Input: part model. Units: mm. Frame: model coordinates. A direction names the side the tool comes from. Coordinates: 2 decimals unless noted, no trailing zeros. Order: outer loops, then holes, each group sorted by start corner. A loop starts at its lowest first (then second) coordinate and runs counter-clockwise, first axis right, second up. Notation, with made-up numbers: (34.5, 75.5) - (81.5, 75.5) arc R20 ccw to (81.5, 86.5) - close; hole circle Ø10 at (23, -8). An arc over 180 degrees is marked (long way). Use a Markdown table: item, result. Add a question column.
from build123d import *
from OCP.BRepFilletAPI import BRepFilletAPI_MakeChamfer

# Parameters (mm, degrees)
EXTRUDE_1_DEPTH     = 131
EXTRUDE_2_DEPTH     = 116
CUT_EXTRUDE_1_REACH = 148.45
CUT_EXTRUDE_2_REACH = 148.994
EXTRUDE_3_DEPTH     = 134
CUT_EXTRUDE_3_DEPTH = 67
EXTRUDE_4_DEPTH     = 11
EXTRUDE_START       = -33.5
EXTRUDE_5_DEPTH     = 67
EXTRUDE_6_DEPTH     = 2
EXTRUDE_7_DEPTH     = 20
EXTRUDE_8_DEPTH     = 10
EXTRUDE_9_DEPTH     = 10
CUT_EXTRUDE_4_REACH = 246.491
SKETCH_16_W         = 5.440253517
SKETCH_16_H         = 47
CUT_EXTRUDE_5_DEPTH = 219.790404517
EXTRUDE_10_DEPTH    = 15
CUT_EXTRUDE_6_DEPTH = 15
EXTRUDE_15_DEPTH    = 77
SKETCH_23_R         = 7
SKETCH_23_R_2       = 4.5
EXTRUDE_16_DEPTH    = 3
CHAMFER_1_SIZE      = 3
CHAMFER_1_SIZE_2    = 1.732050808
CHAMFER_2_SIZE      = 3
CHAMFER_2_SIZE2     = 1.907428497


# Read off the part's stored shape, not the designer's step: 凸台-拉伸5
with BuildPart() as part:
    # 草图1 → 凸台-拉伸1 (new body)
    with BuildSketch(Plane.XY):
        Polygon((0, 0), (3, 20), (39, 20), (42, 0), (39, -35), (3, -35), align=None)
    extrude(amount=-EXTRUDE_1_DEPTH)

    # 草图2 → 凸台-拉伸2 (add)
    with BuildSketch(Plane.XY.offset(-15)):
        Polygon((-2, 24.7), (-4.8, 0.2), (-4.8, -5.8), (-2, -40.3), (21, -40.3), (21, -35), (3, -35), (0, 0), (3, 20), (21, 20), (21, 24.7), align=None)
        Polygon((44, 24.7), (21, 24.7), (21, 20), (39, 20), (42, 0), (39, -35), (21, -35), (21, -40.3), (44, -40.3), (46.8, -5.8), (46.8, 0.2), align=None)
    extrude(amount=-EXTRUDE_2_DEPTH)

    # 切除-拉伸1: up to this plane
    cut_extrude_1_end = Plane(origin=(3, -35, -131), z_dir=(-0.996346649041751, -0.08540114134643588, 0))
    # 草图3 → 切除-拉伸1 (cut, up to the surface)
    with BuildSketch(Plane.ZY.offset(4.8), mode=Mode.PRIVATE) as cut_extrude_1_sk1:
        Polygon((-131, -40.3), (-131, -10.092413278), (-95, -40.3), align=None)
    cut_extrude_1_tool1 = split(extrude(cut_extrude_1_sk1.sketch, amount=-CUT_EXTRUDE_1_REACH, mode=Mode.PRIVATE), bisect_by=cut_extrude_1_end, keep=Keep.BOTH, mode=Mode.PRIVATE)
    add(cut_extrude_1_tool1.solids().sort_by_distance((-4.8, -30.230804, -119))[0], mode=Mode.SUBTRACT)
    # 草图3 → 切除-拉伸1 (cut, up to the surface)
    with BuildSketch(Plane.ZY.offset(4.8), mode=Mode.PRIVATE) as cut_extrude_1_sk2:
        Polygon((-62, -40.3), (-30.5, -8.8), (-15, -8.8), (-15, -40.3), align=None)
    cut_extrude_1_tool2 = split(extrude(cut_extrude_1_sk2.sketch, amount=-CUT_EXTRUDE_1_REACH, mode=Mode.PRIVATE), bisect_by=cut_extrude_1_end, keep=Keep.BOTH, mode=Mode.PRIVATE)
    add(cut_extrude_1_tool2.solids().sort_by_distance((-4.8, -27.196, -31.948))[0], mode=Mode.SUBTRACT)

    # 切除-拉伸2: up to this plane
    cut_extrude_2_end = Plane(origin=(42, 0, -131), z_dir=(0.996346649041751, -0.08540114134643569, 0))
    # 草图4 → 切除-拉伸2 (cut, up to the surface)
    with BuildSketch(Plane(origin=(46.8, 0, 0), x_dir=(0, 0, -1), z_dir=(1, 0, 0)), mode=Mode.PRIVATE) as cut_extrude_2_sk1:
        Polygon((15, -8.919073988), (15, -40.419073988), (62, -40.419073988), (30.5, -8.919073988), align=None)
    cut_extrude_2_tool1 = split(extrude(cut_extrude_2_sk1.sketch, amount=CUT_EXTRUDE_2_REACH, dir=(-0.996346649042, 0.085401141346, 0), mode=Mode.PRIVATE), bisect_by=cut_extrude_2_end, keep=Keep.BOTH, mode=Mode.PRIVATE)
    add(cut_extrude_2_tool1.solids().sort_by_distance((46.8, -27.315074, -31.948))[0], mode=Mode.SUBTRACT)

    # 草图6 → 凸台-拉伸3 (add)
    with BuildSketch(Plane.XY.offset(-11)):
        Polygon((-9, 29.7), (1, 24.7), (41, 24.7), (51, 29.7), (51, 44.7), (41, 49.7), (1, 49.7), (-9, 44.7), align=None)
    extrude(amount=-EXTRUDE_3_DEPTH)

    # 草图7 → 切除-拉伸3 (cut, symmetric)
    with BuildSketch(Plane.ZY.offset(4.8)):
        Polygon((-95, -40.3), (-131, -40.3), (-131, -9.728583388), align=None)
        Polygon((-145, 24.7), (-135, 49.7), (-145, 49.7), align=None)
    extrude(amount=CUT_EXTRUDE_3_DEPTH, both=True, mode=Mode.SUBTRACT)

    # 草图9 → 凸台-拉伸4 (add)
    with BuildSketch(Plane.XY.offset(-11)):
        Polygon((3.5, 45.7), (3.5, 28.7), (8.5, 26.2), (33.5, 26.2), (38.5, 28.7), (38.5, 45.7), (33.5, 48.2), (8.5, 48.2), align=None)
    extrude(amount=EXTRUDE_4_DEPTH)

    # 凸台-拉伸5 outline → 凸台-拉伸5 (add)
    with BuildSketch(Plane.ZY.offset(-21).offset(EXTRUDE_START)):
        with BuildLine():
            Line((-118.5, 35.555969457), (-83.798221281, -5.8))
            ThreePointArc((-83.798221281, -5.8), (-66.915700425, -24.400324924), (-42.17780049, -20.038226285))
            ThreePointArc((-42.17780049, -20.038226285), (-40.182635106, -18.251941452), (-38.381793618, -16.269905038))
            ThreePointArc((-38.381793618, -16.269905038), (-34.014561818, -8.544330565), (-32.5, 0.2))
            Line((-32.5, 0.2), (-32.5, 54.2))
            Line((-32.5, 54.2), (-118.5, 54.2))
            Line((-118.5, 54.2), (-118.5, 35.555969457))
        make_face()
    extrude(amount=EXTRUDE_5_DEPTH)

    # 草图11 → 凸台-拉伸6 (add)
    with BuildSketch(Plane.ZY.offset(12.5)):
        with BuildLine():
            Line((-84.5, 9.7), (-96.804265564, 9.7))
            Line((-96.804265564, 9.7), (-83.798221281, -5.8))
            ThreePointArc((-83.798221281, -5.8), (-66.915700425, -24.400324924), (-42.17780049, -20.038226285))
            ThreePointArc((-42.17780049, -20.038226285), (-40.182635106, -18.251941452), (-38.381793618, -16.269905038))
            ThreePointArc((-38.381793618, -16.269905038), (-34.014561818, -8.544330565), (-32.5, 0.2))
            Line((-32.5, 0.2), (-32.5, 9.7))
            ThreePointArc((-32.5, 9.7), (-58.5, 35.7), (-84.5, 9.7))
        make_face()
    extrude_6 = extrude(amount=EXTRUDE_6_DEPTH)

    # 镜向1: 凸台-拉伸6 across plane
    add(extrude_6.mirror(Plane.ZY.offset(-21)))

    # 草图12 → 凸台-拉伸7 (add)
    with BuildSketch(Plane(origin=(0, 54.2, 0), x_dir=(1, 0, 0), z_dir=(0, 1, 0))):
        Polygon((21, 100), (-6.5, 100), (-6.5, 32.5), (48.5, 32.5), (48.5, 100), align=None)
    extrude(amount=EXTRUDE_7_DEPTH)

    # 草图13 → 凸台-拉伸8 (add)
    with BuildSketch(Plane.ZY.offset(6.5)):
        Polygon((-95, 62.2), (-99.448556281, 147.083510454), (-88.463631398, 147.659205973), (-84.015075118, 62.775695519), align=None)
    extrude(amount=EXTRUDE_8_DEPTH)

    # 草图14 → 凸台-拉伸9 (add)
    with BuildSketch(Plane(origin=(48.5, 0, 0), x_dir=(0, 0, -1), z_dir=(1, 0, 0))):
        Polygon((84.613797545, 74.2), (95.628893351, 74.2), (99.448556281, 147.083510454), (88.463631398, 147.659205973), align=None)
        Polygon((84.015075118, 62.775695519), (95, 62.2), (95.628893351, 74.2), (84.613797545, 74.2), align=None)
    extrude(amount=EXTRUDE_9_DEPTH)

    # 切除-拉伸4: up to this plane
    cut_extrude_4_end = Plane(origin=(-16.436947072, -34.998764239, 0), z_dir=(-0.08540114134643567, -0.996346649041751, 0))
    # 草图16 → 切除-拉伸4 (cut, up to the surface)
    with BuildSketch(Plane.XZ.offset(40.3), mode=Mode.PRIVATE) as cut_extrude_4_sk1:
        with Locations((41.279873241, -38.5)):
            Rectangle(SKETCH_16_W, SKETCH_16_H)
    cut_extrude_4_tool1 = split(extrude(cut_extrude_4_sk1.sketch, amount=-CUT_EXTRUDE_4_REACH, mode=Mode.PRIVATE), bisect_by=cut_extrude_4_end, keep=Keep.BOTH, mode=Mode.PRIVATE)
    add(cut_extrude_4_tool1.solids().sort_by_distance((41.279873, -40.3, -38.5))[0], mode=Mode.SUBTRACT)

    # 草图17 → 切除-拉伸5 (cut, through all)
    with BuildSketch(Plane.ZY.offset(12.5)):
        Polygon((-15, -40.3), (-15, -35), (-56.7, -35), (-62, -40.3), align=None)
    extrude(amount=-CUT_EXTRUDE_5_DEPTH, mode=Mode.SUBTRACT)

    # 草图18 → 凸台-拉伸10 (add)
    with BuildSketch(Plane.XY):
        with BuildLine():
            Line((16.069933514, -1.66230637), (18.041960108, -13.328973037))
            ThreePointArc((18.041960108, -13.328973037), (21, -15.828973037), (23.958039892, -13.328973037))
            Line((23.958039892, -13.328973037), (25.930066486, -1.66230637))
            ThreePointArc((25.930066486, -1.66230637), (21, 4.171026963), (16.069933514, -1.66230637))
        make_face()
    extrude(amount=EXTRUDE_10_DEPTH)

    # 草图20 → 切除-拉伸6 (cut)
    with BuildSketch(Plane.XY.offset(15)):
        with BuildLine():
            Line((17.055946811, -1.495639704), (19.027973406, -13.16230637))
            ThreePointArc((19.027973406, -13.16230637), (21, -14.828973037), (22.972026594, -13.16230637))
            Line((22.972026594, -13.16230637), (24.944053189, -1.495639704))
            ThreePointArc((24.944053189, -1.495639704), (21, 3.171026963), (17.055946811, -1.495639704))
        make_face()
    extrude(amount=-CUT_EXTRUDE_6_DEPTH, mode=Mode.SUBTRACT)

    # 草图21 → 凸台-拉伸15 (add)
    with BuildSketch(Plane.XY.offset(15)):
        with BuildLine():
            Line((13.111893623, -2.16230637), (15.083920217, -13.828973037))
            ThreePointArc((15.083920217, -13.828973037), (21, -18.828973037), (26.916079783, -13.828973037))
            Line((26.916079783, -13.828973037), (28.888106377, -2.16230637))
            ThreePointArc((28.888106377, -2.16230637), (21, 7.171026963), (13.111893623, -2.16230637))
        make_face()
    extrude(amount=EXTRUDE_15_DEPTH)

    # 草图23 → 凸台-拉伸16 (add)
    with BuildSketch(Plane.XY.offset(92)):
        with Locations((21, -0.828973037)):
            Circle(SKETCH_23_R)
        with Locations((21, -12.828973037)):
            Circle(SKETCH_23_R_2)
    extrude(amount=EXTRUDE_16_DEPTH)

    # 倒角1
    chamfer_1_edges_1 = [part.edges().sort_by_distance(p)[0] for p in [
        (14, -0.828973037, 95),
    ]]
    chamfer_1_side_1 = [part.faces().sort_by_distance(p)[0] for p in [
        (14, -0.828973037, 94.965358984),
    ]]
    chamfer_1_edges_2 = [part.edges().sort_by_distance(p)[0] for p in [
        (16.5, -12.828973037, 95),
    ]]
    chamfer_1_side_2 = [part.faces().sort_by_distance(p)[0] for p in [
        (16.5, -12.828973037, 94.965358984),
    ]]
    chamfer_1 = BRepFilletAPI_MakeChamfer(part.part.solid().wrapped)
    for e in chamfer_1_edges_1:
        chamfer_1.Add(CHAMFER_1_SIZE - 0.0001, CHAMFER_1_SIZE_2 - 0.0001, e.wrapped, chamfer_1_side_1[0].wrapped)
    for e in chamfer_1_edges_2:
        chamfer_1.Add(CHAMFER_1_SIZE - 0.0001, CHAMFER_1_SIZE_2 - 0.0001, e.wrapped, chamfer_1_side_2[0].wrapped)
    add(Compound.cast(chamfer_1.Shape()), mode=Mode.REPLACE)  # a hair under: the kernel refuses the full size

    # 倒角2: one chamfer whose edges measure the first distance from different faces: ONE call of the kernel's chamfer builder (chamfer() names one face for all edges)
    chamfer_2_edges_1 = [part.edges().sort_by_distance(p)[0] for p in [
        (3, -35, -28.35),
    ]]
    chamfer_2_side_1 = [part.faces().sort_by_distance(p)[0] for p in [
        (21, -35, -28.35),
    ]]
    chamfer_2_edges_2 = [part.edges().sort_by_distance(p)[0] for p in [
        (39, -35, -28.35),
    ]]
    chamfer_2_side_2 = [part.faces().sort_by_distance(p)[0] for p in [
        (40.177893681, -21.257907057, -21.206076587),
    ]]
    chamfer_2 = BRepFilletAPI_MakeChamfer(part.part.solid().wrapped)
    for e in chamfer_2_edges_1:
        chamfer_2.Add(CHAMFER_2_SIZE, CHAMFER_2_SIZE2, e.wrapped, chamfer_2_side_1[0].wrapped)  # the first distance lies on this face
    for e in chamfer_2_edges_2:
        chamfer_2.Add(CHAMFER_2_SIZE, CHAMFER_2_SIZE2, e.wrapped, chamfer_2_side_2[0].wrapped)  # the first distance lies on this face
    add(Compound.cast(chamfer_2.Shape()), mode=Mode.REPLACE)


solid = part.part
1) Pull-direction query (Y, two-part tool) for faces 5 (the flat face through (-12.5, 37, -76)), 6 (the flat face through (43.949, -8.675, -22.858)), 7 (the flat face through (21, 48.2, -6)); classes: pulls with the +Y half, pulls with the -Y half, needs draft (parallel to the pull), parting line crosses it, or undercut.
2) Material intervals for L1, parallel to Y at x = 7, z = -26; L2, parallel to Z at x = 27, y = 16; L3, parallel to Z at x = 40.5, y = 17, sorted ascending.
3) Cut plane A-A (y = 124). Return the cut outline in (x, z), and give its area (3 significant figures).
4) Cut plane B-B (z = 48). Return the cut outline in (x, y), and give its area (3 significant figures).
5) Contact query for flat-ended pins moving along their axis: P1, Ø10, axis at x = 9.5, y = 65.5, coming from the -Z side; P2, Ø12, axis at x = -8.5, y = -19, coming from the -Z side; P3, Ø22, axis at y = 63, z = -57.5, coming from the -X side. Output: stop coordinate, or through.
6) Cut plane C-C (y = 32.5). Return the cut outline in (x, z).
7) Reachability of faces 1 (the flat face through (46.07, 47.165, -21.6)), 2 (the flat face through (48.5, 111, -92)), 3 (the flat face through (-2, -8.8, -23)), 4 (the flat face through (21, 64, -100)) from +Z, -Z, +X, -X, +Y, -Y: full face, straight path, thin tool, end or side. Return the list, or none.
8) Cut plane D-D (z = -104). Return the cut outline in (x, y).
Computed:
| question | item | result |
|---|---|---|
| 1 | face 5 | undercut |
| 1 | face 6 | pulls with the -Y half |
| 1 | face 7 | pulls with the +Y half |
| 2 | L1 | y = -35 to 49.7 |
| 2 | L2 | z = -131 to 0 |
| 2 | L3 | z = -131 to -15 |
| 3 | outline | (-16.5, -98.24) - (-6.5, -98.24) - (-6.5, -87.22) - (-16.5, -87.22) - close; (48.5, -98.24) - (58.5, -98.24) - (58.5, -87.22) - (48.5, -87.22) - close |
| 3 | area | 220 mm2 |
| 4 | outline | (13.11, -2.16) - (15.08, -13.83) arc R6 ccw to (26.92, -13.83) - (28.89, -2.16) arc R8 ccw (long way) to start |
| 4 | area | 327 mm2 |
| 5 | P1 | stops at z = -100 |
| 5 | P2 | stops at z = -124.83 |
| 5 | P3 | stops at x = -12.5 |
| 6 | outline | (-14.5, -71) - (-12.5, -71) - (-12.5, -115.94) - (-9, -115.94) - (-9, -141.88) - (51, -141.88) - (51, -115.94) - (54.5, -115.94) - (54.5, -71) - (56.5, -71) - (56.5, -46) - (54.5, -46) - (54.5, -32.5) - (51, -32.5) - (51, -11) - (38.5, -11) - (38.5, 0) - (3.5, 0) - (3.5, -11) - (-9, -11) - (-9, -32.5) - (-12.5, -32.5) - (-12.5, -46) - (-14.5, -46) - close |
| 7 | face 1 | +Z, +X, +Y |
| 7 | face 2 | +Z, -Z, +Y |
| 7 | face 3 | +Z, -X, -Y |
| 7 | face 4 | -Z, +X, -X, +Y |
| 8 | outline | (-12.5, 18.28) - (-2.73, 18.28) - (-4.8, 0.2) - (-4.8, -5.8) - (-2.62, -32.66) - (44.62, -32.66) - (46.8, -5.8) - (46.8, 0.2) - (44.73, 18.28) - (54.5, 18.28) - (54.5, 54.2) - (-12.5, 54.2) - close |
